Geometry check sheet. Reference: the model listing, model coordinates, mm. A direction names the side the tool comes from. Round coordinates to 2 decimals unless told otherwise and drop trailing zeros. Write each loop counter-clockwise with the first axis right and the second up, starting at its lowest first coordinate (ties: lowest second). Pieces come first, ordered by that corner, then holes. Notation, with made-up numbers: M 40.25,-32 L 57.25,-32 A33 cw 57.25,6 Z; hole C 53,3.25 d1. An arc over 180 degrees is marked long. Answer as CSV lines item,"result". Start each with the question number.
```python
from build123d import *

# Parameters (mm, degrees)
F0_R     = 9.525
F1_DEPTH = 25.4
F3_DEPTH = 25.401
F4_DEPTH = 11.0998
F6_DEPTH = 9.525


with BuildPart() as f1:
    # F0 (on Front) → F1 (new body)
    with BuildSketch(Plane.XZ):
        Circle(F0_R)
    extrude(amount=F1_DEPTH)

    # F2 (on Front) → F3 (cut, through all)
    with BuildSketch(Plane.XZ):
        with BuildLine():
            ThreePointArc((-4.7625, 0), (-3.367596, -3.367596), (0, -4.7625))
            ThreePointArc((0, -4.7625), (3.367596, -3.367596), (4.7625, 0))
            ThreePointArc((4.7625, 0), (3.367596, 3.367596), (0, 4.7625))
            ThreePointArc((0, 4.7625), (-3.367596, 3.367596), (-4.7625, 0))
        make_face()
    extrude(amount=F3_DEPTH, mode=Mode.SUBTRACT)

    # F2 (on Front) → F4 (cut)
    with BuildSketch(Plane.XZ):
        with BuildLine():
            Line((0, -4.7625), (4.7625, -4.7625))
            Line((4.7625, -4.7625), (4.7625, 0))
            ThreePointArc((4.7625, 0), (3.367596, -3.367596), (0, -4.7625))
        make_face()
        with BuildLine():
            Line((-4.7625, -4.7625), (0, -4.7625))
            ThreePointArc((0, -4.7625), (-3.367596, -3.367596), (-4.7625, 0))
            Line((-4.7625, 0), (-4.7625, -4.7625))
        make_face()
        with BuildLine():
            ThreePointArc((0, 4.7625), (3.367596, 3.367596), (4.7625, 0))
            Line((4.7625, 0), (4.7625, 4.7625))
            Line((4.7625, 4.7625), (0, 4.7625))
        make_face()
        with BuildLine():
            Line((-4.7625, 4.7625), (-4.7625, 0))
            ThreePointArc((-4.7625, 0), (-3.367596, 3.367596), (0, 4.7625))
            Line((0, 4.7625), (-4.7625, 4.7625))
        make_face()
    extrude(amount=-F4_DEPTH, mode=Mode.SUBTRACT)

    # F5 (on face) → F6 (cut)
    with BuildSketch(Plane(origin=(0, 0, 0), x_dir=(-1, 0, 0), z_dir=(0, 1, 0))):
        Polygon((0.99988, -7.854919), (7.3025, -3.061538), (6.30262, 4.793382), (-0.99988, 7.854919), (-7.3025, 3.061538), (-6.30262, -4.793382), align=None)
    extrude(amount=-F6_DEPTH, mode=Mode.SUBTRACT)


solid = f1.part
```
1) Mould release check, pull along X, two halves, no side actions. Record for faces 3 (the flat face through (-4.4, -25.4, 2.3)), 4 (the cylindrical face through (-7.559, -12.522, -5.796)), 5 (the flat face through (-4.11, -4.7, -5.49)): released by +X, released by -X, zero draft, split by the parting line, or undercut.
2) Section check C-C, the plane z = 1.25. Record the cut outline in (x, y) (3 decimals), plus the area to 3 significant figures.
3) Access from +Z, -Z, +X, -X, +Y, -Y to the whole of each face (thin tool, end or side, straight path). Record for faces 1 (the flat face through (6.81, -4.7, -0.81)), 2 (the flat face through (-4, 0, -6)).
4) Scan lines: line 1 (X direction, y = -1.75, z = -0.25); line 2 (Z direction, x = -3, y = -10.5); line 3 (Z direction, x = 3.75, y = -23.5). Record each from-to range of solid material in increasing order. Write a range as from..to.
5) Section check B-B, the plane x = 0.5. Record the cut outline in (y, z) (3 decimals), plus the area to 3 significant figures.
6) Go/stop test with flat-tipped pins: pin 1 (4 mm diameter, centred on x = -3.5, y = -2.5, fed in from +Z); pin 2 (3 mm diameter, centred on x = 5.5, z = 2, fed in from +Y) (3 decimals); pin 3 (10 mm diameter, centred on y = -10, z = 7, fed in from -X). Record where each tip stops, or that it passes through.
7) Section check D-D, the plane z = 6.75. Record the cut outline in (x, y) (3 decimals), plus the area to 3 significant figures.
Results:
1,face 3,"zero draft"
1,face 4,"split by the parting line"
1,face 5,"undercut"
2,outline,"M -9.443,-25.4 L -4.596,-25.4 L -4.596,-9.525 L -6.754,-9.525 L -6.754,0 L -9.443,0 Z; M 4.596,-25.4 L 9.443,-25.4 L 9.443,0 L 7.072,0 L 7.072,-9.525 L 4.596,-9.525 Z"
2,area,"202 mm^2"
3,face 1,"+Y"
3,face 2,"+Z, -Z, +X, -X, +Y"
4,line 1,"x = -9.52..-6.94, 6.88..9.52"
4,line 2,"z = -9.04..-3.7, 3.7..9.04"
4,line 3,"z = -8.76..-2.94, 2.94..8.76"
5,outline,"M -25.4,-9.512 L 0,-9.512 L 0,-7.226 L -9.525,-7.226 L -9.525,-4.736 L -25.4,-4.736 Z; M -25.4,4.736 L -9.525,4.736 L -9.525,7.645 L 0,7.645 L 0,9.512 L -25.4,9.512 Z"
5,area,"191 mm^2"
6,pin 1,"stops at z = 9.41"
6,pin 2,"stops at y = -9.525"
6,pin 3,"stops at x = -9.31"
7,outline,"M -6.72,-25.4 L 6.72,-25.4 L 6.72,0 L 2.453,0 L 2.453,-9.525 L -1.636,-9.525 L -1.636,0 L -6.72,0 Z"
7,area,"302 mm^2"
